The drawing under review shows one solid part. Ordinate dimensions are in mm from its lowest x, y, z. Give positions to 0.01 mm unless a question says otherwise; leave off trailing zeros. Loops run counter-clockwise (first coordinate to the right, second up) from the corner with the lowest first, then second, coordinate; pieces in that order, holes last.
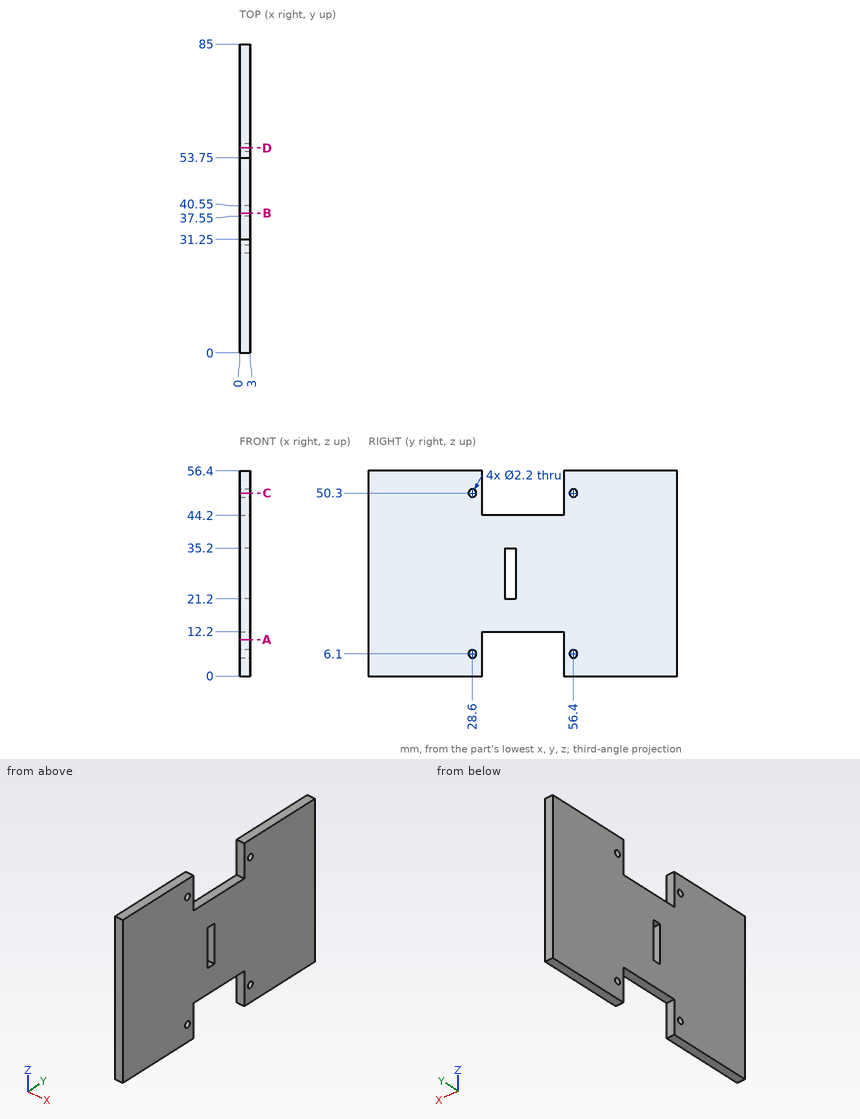
Item 1: Take a section at B-B on y = 38.5. Give the boundary of the cut face in (x, z).
Answer:
outline: (0, 12.2) - (3, 12.2) - (3, 21.2) - (0, 21.2) - close; (0, 35.2) - (3, 35.2) - (3, 44.2) - (0, 44.2) - close
Item 2: Take a section at A-A on z = 10. Give the boundary of the cut face in (x, y), and give its area (4 significant figures).
Answer:
outline: (0, 0) - (3, 0) - (3, 31.25) - (0, 31.25) - close; (0, 53.75) - (3, 53.75) - (3, 85) - (0, 85) - close
area: 187.5 mm2
Item 3: Take a section at D-D on y = 56.4. Give the boundary of the cut face in (x, z).
Answer:
outline: (0, 0) - (3, 0) - (3, 5) - (0, 5) - close; (0, 7.2) - (3, 7.2) - (3, 49.2) - (0, 49.2) - close; (0, 51.4) - (3, 51.4) - (3, 56.4) - (0, 56.4) - close
Item 4: Clearance check with flat-ended pins moving along their axes: pin 1 Ø1.8 at (y, z) = (28.6, 6.1) entering from -X (3 decimals); pin 2 Ø1.5 at (x, y) = (2, 39.5) entering from +Z; pin 3 Ø0.9 at (x, y) = (1, 39) entering from -Z. State where each tip first meets the part, or that it passes through.
Answer:
pin 1: passes through
pin 2: stops at z = 44.2
pin 3: stops at z = 12.2
Item 5: For L1, parallel to Y at x = 1.95, z = 6.1; L2, parallel to Y at x = 1.9, z = 54.5; L3, parallel to Y at x = 1.5, z = 7, list the stretches that pass through material, from the lowest coordinate up.
Answer:
L1: y = 0 to 27.5, 29.7 to 31.25, 53.75 to 55.3, 57.5 to 85
L2: y = 0 to 31.25, 53.75 to 85
L3: y = 0 to 27.97, 29.23 to 31.25, 53.75 to 55.77, 57.03 to 85
Item 6: Take a section at C-C on z = 50.3. Give the boundary of the cut face in (x, y).
Answer:
outline: (0, 0) - (3, 0) - (3, 27.5) - (0, 27.5) - close; (0, 29.7) - (3, 29.7) - (3, 31.25) - (0, 31.25) - close; (0, 53.75) - (3, 53.75) - (3, 55.3) - (0, 55.3) - close; (0, 57.5) - (3, 57.5) - (3, 85) - (0, 85) - close
